For this review, use the dimensioned drawing (mm, ordinates from the lowest corner) and the shaded views. A direction names the side the tool comes from. Round coordinates to 2 decimals unless told otherwise and drop trailing zeros. Order: outer loops, then holes, each group sorted by start corner. A loop starts at its lowest first (then second) coordinate and runs counter-clockwise, first axis right, second up. Notation, with made-up numbers: M 43.5,69.25 L 72.5,69.25 A18 cw 72.5,94.25 Z; hole C 9,34 d2. An arc over 180 degrees is marked long. Use a Markdown table: item, result. Add a question column.
1. Consider section D-D on y = 35.5. State the section outline as (x, z) points.
2. Consider section C-C on x = 43.15. State the section outline as (y, z) points (3 decimals), then the cut area to 3 significant figures.
3. Consider section B-B on y = 21. State the section outline as (x, z) points (3 decimals), then the cut area to 3 significant figures.
4. Consider section A-A on x = 14.25. State the section outline as (y, z) points, then the cut area to 3 significant figures.
5. Insertion check: P1, Ø8, axis at x = 8.5, y = 11.5, coming from the +Z side; P2, Ø6, axis at x = 48.5, z = 19, coming from the -Y side; P3, Ø3, axis at x = 8, y = 12.5, coming from the +Z side. Each pin has a flat end and moves straight along its axis. Give the tip position at first contact, or say it passes through.
6. To check wall thickness, follow probe 1 along Z at (x, y) = (21, 21.5); probe 2 along Z at (x, y) = (10.5, 8.5); probe 3 along X at (y, z) = (29, 21.5). State the ranges of each line that lie inside material, in increasing order.
7. For the marked faces 1, 2 and 3, list the 3-axis set-ups (+Z, -Z, +X, -X, +Y, -Y) from which the entire face can be reached by the end or side of a thin tool; tool diameter is ignored.
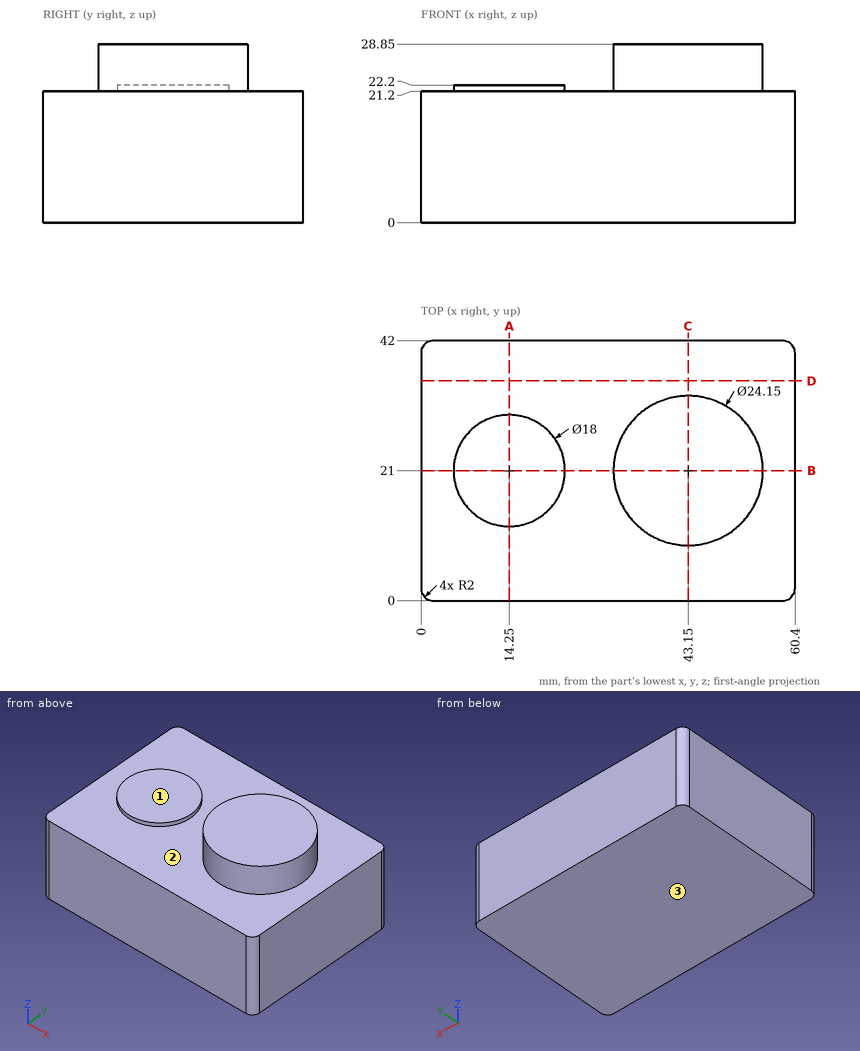
Answer block:
| question | item | result |
|---|---|---|
| 1 | outline | M 0,0 L 60.4,0 L 60.4,21.2 L 0,21.2 Z |
| 2 | outline | M 0,0 L 42,0 L 42,21.2 L 33.075,21.2 L 33.075,28.85 L 8.925,28.85 L 8.925,21.2 L 0,21.2 Z |
| 2 | area | 1,080 mm^2 |
| 3 | outline | M 0,0 L 60.4,0 L 60.4,21.2 L 55.225,21.2 L 55.225,28.85 L 31.075,28.85 L 31.075,21.2 L 23.25,21.2 L 23.25,22.2 L 5.25,22.2 L 5.25,21.2 L 0,21.2 Z |
| 3 | area | 1,480 mm^2 |
| 4 | outline | M 0,0 L 42,0 L 42,21.2 L 30,21.2 L 30,22.2 L 12,22.2 L 12,21.2 L 0,21.2 Z |
| 4 | area | 908 mm^2 |
| 5 | P1 | z = 22.2 |
| 5 | P2 | y = 0 |
| 5 | P3 | z = 21.2 |
| 6 | probe 1 | 0 to 22.2 |
| 6 | probe 2 | 0 to 21.2 |
| 6 | probe 3 | 10.13 to 18.37, 34.11 to 52.19 |
| 7 | face 1 | +Z, -X, +Y, -Y |
| 7 | face 2 | +Z |
| 7 | face 3 | -Z, +X, -X, +Y, -Y |
